Source: CAD feature listing. Evaluate the final solid. Frame: model axes, mm. A direction names the side the tool comes from. Coordinates: 2 decimals unless noted, no trailing zeros. Loops run counter-clockwise (first coordinate to the right, second up) from the corner with the lowest first, then second, coordinate; pieces in that order, holes last.
Item 1: Reachability of faces 4 (the flat face through (-12.082, -12.283, -14.79)), 5 (the flat face through (12, 1, -30)) from +Z, -Z, +X, -X, +Y, -Y: full face, straight path, thin tool, end or side. Return the list, or none.
Item 2: Section query A-A, the plane y = 55. Return the cut outline in (x, z), then the cut area to 3 significant figures.
Item 3: Section query C-C, the plane x = 33. Return the cut outline in (y, z), then the cut area to 3 significant figures.
Item 4: Pull-direction query (Y, two-part tool) for faces 1 (the flat face through (12, 1, 0)), 2 (the flat face through (12.283, -12.082, -14.79)), 3 (the cylindrical face through (-59.94, 2.64, -14.79)); classes: +Y half, -Y half, draft (parallel to the pull), parting line (faces both ways), or undercut.
Item 5: Line query: probe 1 along X at (y, z) = (16.5, -18.25); probe 2 along X at (y, z) = (25.5, -15.25); probe 3 along Y at (x, z) = (-9.5, -24.25). Output: solid intervals per line, ascending.
Item 6: Section query D-D, the plane y = 12. Return the cut outline in (x, z).
Item 7: Pin query (flat end, axial travel): pin 1 Ø4 at (x, y) = (24.18, 0) entering from -Z; pin 2 Ø12 at (y, z) = (-8.5, -4.5) entering from -X; pin 3 Ø3 at (y, z) = (-27.5, -21.5) entering from -X; pin 4 Ø6 at (x, z) = (14.5, -8) entering from -Y. Return the tip coordinate at first contact, or that it passes through.
```python
from build123d import *

# Parameters (mm, degrees)
SKETCH6_R                 = 29
SKETCH6_R_2               = 20
INNER_RING_DEPTH          = 30
MOTOR_CONNECTOR_CUT_DEPTH = 30
M3_HOLES_DEPTH            = 38
M3_HOLES_DEPTH_BACK       = 100
SKETCH8_R                 = 2.5
MIDDLE_PATTERN_DEPTH      = 30
SKETCH9_R                 = 60
SKETCH9_R_2               = 50
SKETCH9_R_3               = 2.5
BOSS_EXTRUDE1_DEPTH       = 30
BOSS_EXTRUDE2_DEPTH       = 30


with BuildPart() as part:
    # Sketch6 → Inner Ring (new body)
    with BuildSketch(Plane.XY):
        Circle(SKETCH6_R)
        Circle(SKETCH6_R_2, mode=Mode.SUBTRACT)
    extrude(amount=-INNER_RING_DEPTH)

    # Sketch7 → Motor Connector Cut (add)
    with BuildSketch(Plane.XY):
        with BuildLine():
            ThreePointArc((20, 0), (19.840593925, 2.52008585), (19.364916731, 5))
            Line((19.364916731, 5), (9.999996731, 5))
            Line((9.999996731, 5), (9.999996731, -5))
            Line((9.999996731, -5), (19.364916731, -5))
            ThreePointArc((19.364916731, -5), (19.840593925, -2.52008585), (20, 0))
        make_face()
        with BuildLine():
            ThreePointArc((5, 19.364916731), (0, 20), (-5, 19.364916731))
            Line((-5, 19.364916731), (-5, 9.999996731))
            Line((-5, 9.999996731), (5, 9.999996731))
            Line((5, 9.999996731), (5, 19.364916731))
        make_face()
        with BuildLine():
            Line((-9.999996731, -5), (-9.999996731, 5))
            Line((-9.999996731, 5), (-19.364916731, 5))
            ThreePointArc((-19.364916731, 5), (-20, 0), (-19.364916731, -5))
            Line((-19.364916731, -5), (-9.999996731, -5))
        make_face()
        with BuildLine():
            Line((-5, -9.999996731), (-5, -19.364916731))
            ThreePointArc((-5, -19.364916731), (0, -20), (5, -19.364916731))
            Line((5, -19.364916731), (5, -9.999996731))
            Line((5, -9.999996731), (-5, -9.999996731))
        make_face()
    extrude(amount=-MOTOR_CONNECTOR_CUT_DEPTH)

    # Sketch8 → M3 Holes (cut, two sides: drawn at the far end of the back side and taken through both)
    with BuildSketch(Plane.XY.offset(-M3_HOLES_DEPTH_BACK)):
        with Locations((0, 24.182458366)):
            Circle(SKETCH8_R)
        with Locations((24.182458366, 0)):
            Circle(SKETCH8_R)
        with Locations((0, -24.182458366)):
            Circle(SKETCH8_R)
        with Locations((-24.182458366, 0)):
            Circle(SKETCH8_R)
    extrude(amount=M3_HOLES_DEPTH + M3_HOLES_DEPTH_BACK, mode=Mode.SUBTRACT)

    # Sketch10 → Middle Pattern (add)
    with BuildSketch(Plane.XY):
        with BuildLine():
            ThreePointArc((28.607215414, 4.756808408), (26.539406056, -11.690163651), (15.800414568, -24.317625284))
            ThreePointArc((15.800414568, -24.317625284), (11.745224483, -41.595013937), (-4.095362954, -49.596795923))
            ThreePointArc((-4.095362954, -49.596795923), (-2.057581903, -49.898955876), (-2.31e-07, -50))
            ThreePointArc((-2.31e-07, -50), (19.134171511, -46.19397667), (35.355339059, -35.355339059))
            ThreePointArc((35.355339059, -35.355339059), (42.321804958, -13.559663633), (28.607215414, 4.756808408))
        make_face()
        with BuildLine():
            ThreePointArc((24.317625284, 15.800414568), (41.595013937, 11.745224483), (49.596795923, -4.095362954))
            ThreePointArc((49.596795923, -4.095362954), (49.898955887, -2.057581788), (50, 0))
            ThreePointArc((50, 0), (46.193976626, 19.134171618), (35.355339059, 35.355339059))
            ThreePointArc((35.355339059, 35.355339059), (13.559663633, 42.321804958), (-4.756808408, 28.607215414))
            ThreePointArc((-4.756808408, 28.607215414), (11.690163651, 26.539406056), (24.317625284, 15.800414568))
        make_face()
        with BuildLine():
            ThreePointArc((8.201394106, 49.322785148), (-15.267827902, 47.611904301), (-35.355339044, 35.355339075))
            ThreePointArc((-35.355339044, 35.355339075), (-42.32180496, 13.559663644), (-28.607215414, -4.756808408))
            ThreePointArc((-28.607215414, -4.756808408), (-26.539406056, 11.690163651), (-15.800414568, 24.317625284))
            ThreePointArc((-15.800414568, 24.317625284), (-10.393277189, 43.149392225), (8.201394106, 49.322785148))
        make_face()
        with BuildLine():
            ThreePointArc((4.756808408, -28.607215414), (-11.690163651, -26.539406056), (-24.317625284, -15.800414568))
            ThreePointArc((-24.317625284, -15.800414568), (-41.595013937, -11.745224483), (-49.596795923, 4.095362954))
            ThreePointArc((-49.596795923, 4.095362954), (-49.898955887, 2.057581788), (-50, 0))
            ThreePointArc((-50, 0), (-46.193976566, -19.134171762), (-35.355338839, -35.35533928))
            ThreePointArc((-35.355338839, -35.35533928), (-13.559663479, -42.321804932), (4.756808408, -28.607215414))
        make_face()
    extrude(amount=-MIDDLE_PATTERN_DEPTH)



with BuildPart() as body_2:
    # Sketch9 → Boss-Extrude1 (new body)
    with BuildSketch(Plane.XY):
        Circle(SKETCH9_R)
        Circle(SKETCH9_R_2, mode=Mode.SUBTRACT)
        with Locations((0, 55)):
            Circle(SKETCH9_R_3, mode=Mode.SUBTRACT)
        with Locations((-38.890872965, 38.890872965)):
            Circle(SKETCH9_R_3, mode=Mode.SUBTRACT)
        with Locations((-55, 0)):
            Circle(SKETCH9_R_3, mode=Mode.SUBTRACT)
        with Locations((-38.890872965, -38.890872965)):
            Circle(SKETCH9_R_3, mode=Mode.SUBTRACT)
        with Locations((0, -55)):
            Circle(SKETCH9_R_3, mode=Mode.SUBTRACT)
        with Locations((38.890872965, -38.890872965)):
            Circle(SKETCH9_R_3, mode=Mode.SUBTRACT)
        with Locations((55, 0)):
            Circle(SKETCH9_R_3, mode=Mode.SUBTRACT)
        with Locations((38.890872965, 38.890872965)):
            Circle(SKETCH9_R_3, mode=Mode.SUBTRACT)
    extrude(amount=-BOSS_EXTRUDE1_DEPTH)


with BuildPart() as part_1:
    add(part.part)

    add(body_2.part)  # Boss-Extrude2 merges body 2
    # Sketch11 → Boss-Extrude2 (add)
    with BuildSketch(Plane.XY):
        with BuildLine():
            Line((-19.364916731, 5), (-5, 19.364916731))
            ThreePointArc((-5, 19.364916731), (-14.142135624, 14.142135624), (-19.364916731, 5))
        make_face()
        with BuildLine():
            Line((5, 19.364916731), (19.364916731, 5))
            ThreePointArc((19.364916731, 5), (14.142135624, 14.142135624), (5, 19.364916731))
        make_face()
        with BuildLine():
            Line((19.364916731, -5), (5, -19.364916731))
            ThreePointArc((5, -19.364916731), (14.142135624, -14.142135624), (19.364916731, -5))
        make_face()
        with BuildLine():
            Line((-5, -19.364916731), (-19.364916731, -5))
            ThreePointArc((-19.364916731, -5), (-14.142135624, -14.142135624), (-5, -19.364916731))
        make_face()
    extrude(amount=-BOSS_EXTRUDE2_DEPTH)


solid = part_1.part
```
Verdict:
1. face 4: +Z, -Z
1. face 5: -Z, +X, -X, +Y, -Y
2. outline: (-23.98, -30) - (-2.5, -30) - (-2.5, 0) - (-23.98, 0) - close; (2.5, -30) - (23.98, -30) - (23.98, 0) - (2.5, 0) - close
2. area: 1,290 mm2
3. outline: (-50.11, -30) - (2.03, -30) - (2.03, 0) - (-50.11, 0) - close; (15.78, -30) - (37.43, -30) - (37.43, 0) - (15.78, 0) - close; (37.56, -30) - (50.11, -30) - (50.11, 0) - (37.56, 0) - close
3. area: 2,590 mm2
4. face 1: draft
4. face 2: undercut
4. face 3: parting line
5. probe 1: x = -57.69 to -47.2, -42.64 to -7.86, -5 to 5, 7.86 to 57.69
5. probe 2: x = -54.31 to -43.01, -41.42 to -16.01, -13.81 to -2.12, 2.12 to 54.31
5. probe 3: y = -59.24 to -49.09, -41.28 to -14.86, 14.86 to 27.4, 44.03 to 59.24
6. outline: (-58.79, -30) - (-48.54, -30) - (-48.54, 0) - (-58.79, 0) - close; (-42.01, -30) - (-12.36, -30) - (-12.36, 0) - (-42.01, 0) - close; (-5, -30) - (5, -30) - (5, 0) - (-5, 0) - close; (12.36, -30) - (26.4, -30) - (26.4, 0) - (12.36, 0) - close; (41.26, -30) - (58.79, -30) - (58.79, 0) - (41.26, 0) - close
7. pin 1: passes through
7. pin 2: stops at x = -59.95
7. pin 3: stops at x = -54.07
7. pin 4: stops at y = -58.89
